Design review of the part built by this model. Coordinates are the model's own, in mm. A direction names the side the tool comes from. Coordinates: 2 decimals unless noted, no trailing zeros. Write each loop counter-clockwise with the first axis right and the second up, starting at its lowest first coordinate (ties: lowest second). Pieces come first, ordered by that corner, then holes. Notation, with made-up numbers: (12, -15.75) -> (58, -15.75) arc R21 cw to (58, 15.25) -> close; hole circle Ø11 at (-30.75, -11). An arc over 180 degrees is marked (long way). Return JSON: item names as keys, results as strings. Group by question number.
from build123d import *

# Parameters (mm, degrees)
BOSS_EXTRUDE1_DEPTH = 50.8
SKETCH2_R           = 2.54
CUT_EXTRUDE1_DEPTH  = 73.955945611
SKETCH3_R           = 3.175
CUT_EXTRUDE2_DEPTH  = 73.955945611
CHAMFER1_SIZE       = 2.54


with BuildPart() as part:
    # Sketch1 → Boss-Extrude1 (new body)
    with BuildSketch(Plane(origin=(0, 0, 0), x_dir=(0, 0, -1), z_dir=(1, 0, 0))):
        with BuildLine():
            Line((0, 1.5875), (0, 50.8))
            Line((0, 50.8), (1.5875, 50.8))
            Line((1.5875, 50.8), (1.5875, 3.175))
            ThreePointArc((1.5875, 3.175), (2.052467985, 2.052467985), (3.175, 1.5875))
            Line((3.175, 1.5875), (12.7, 1.5875))
            Line((12.7, 1.5875), (12.7, 0))
            Line((12.7, 0), (1.5875, 0))
            ThreePointArc((1.5875, 0), (0.464967985, 0.464967985), (0, 1.5875))
        make_face()
    extrude(amount=BOSS_EXTRUDE1_DEPTH)

    # Sketch2 → Cut-Extrude1 (cut, through all)
    with BuildSketch(Plane.XZ):
        with Locations(Location((38.1, -6.35, 0), (0, 0, 270))):
            Circle(SKETCH2_R)
        with Locations(Location((12.7, -6.35, 0), (0, 0, 270))):
            Circle(SKETCH2_R)
    extrude(amount=-CUT_EXTRUDE1_DEPTH, mode=Mode.SUBTRACT)

    # Sketch3 → Cut-Extrude2 (cut, through all)
    with BuildSketch(Plane.XY):
        with Locations((25.4, 25.4)):
            Circle(SKETCH3_R)
    extrude(amount=-CUT_EXTRUDE2_DEPTH, mode=Mode.SUBTRACT)

    # Chamfer1
    chamfer1_edges = [part.edges().sort_by_distance(p)[0] for p in [
        (0, 50.8, -0.79375),
        (50.8, 0.79375, -12.7),
        (50.8, 50.8, -0.79375),
        (0, 0.79375, -12.7),
    ]]
    chamfer(chamfer1_edges, length=CHAMFER1_SIZE)


solid = part.part
Q1. We need section A-A on z = -6.35. Write out the cut boundary in (x, y), plus the area to 3 significant figures.
Q2. Wall thickness on L1, parallel to X at y = 1.1, z = -6.35; L2, parallel to Z at x = 40, y = 17.5; L3, parallel to Y at x = 34, z = -5.5: over which ranges is each line inside the solid? List them lowest first.
Q3. The part is to be moulded in two halves that separate along X. For faces 3 (the flat face through (50.8, 21, -1)), 4 (the cylindrical face through (15.22, 0.78, -6.02)), 5 (the flat face through (1.29, 0.8, -11.45)), say which applies: +X half, -X half, draft (parallel to the pull), parting line (faces both ways), or undercut.
Q4. For P1, Ø1, axis at x = 35, z = -8.5, coming from the +Y side; P2, Ø4.5, axis at x = 38.1, z = -6.35, coming from the -Y side; P3, Ø14.5, axis at x = 17, y = 37, coming from the -Z side, all flat-tipped, find the tip position at first contact; note any pin that passes through.
Q5. We need section D-D on x = 38.1. Write out the cut boundary in (y, z) (1 decimal), plus the area to 3 significant figures.
Q6. We need section C-C on y = 25.4. Write out the cut boundary in (x, z) (1 decimal).
Q7. For faces 1 (the flat face through (25, 22, -1.588)), 2 (the flat face through (25, 50.8, -1)), list the 3-axis set-ups (+Z, -Z, +X, -X, +Y, -Y) from which the entire face can be reached by the end or side of a thin tool; tool diameter is ignored.
Q8. We need section B-B on x = 25.4. Write out the cut boundary in (y, z) (1 decimal), plus the area to 3 significant figures.
Findings below:
{
 "1": {"outline": "(0, 0) -> (10.16, 0) -> (10.16, 1.59) -> (0, 1.59) -> close; (15.24, 0) -> (35.56, 0) -> (35.56, 1.59) -> (15.24, 1.59) -> close; (40.64, 0) -> (50.8, 0) -> (50.8, 1.59) -> (40.64, 1.59) -> close", "area": "64.5 mm^2"},
 "2": {"L1": "x = 0 to 10.16, 15.24 to 35.56, 40.64 to 50.8", "L2": "z = -1.59 to 0", "L3": "y = 0 to 1.59"},
 "3": {"face 3": "+X half", "face 4": "undercut", "face 5": "-X half"},
 "4": {"P1": "stops at y = 1.59", "P2": "passes through", "P3": "stops at z = -1.59"},
 "5": {"outline": "(0, -12.7) -> (1.6, -12.7) -> (1.6, -8.9) -> (0, -8.9) -> close; (0, -3.8) -> (1.6, -3.8) -> (1.6, -3.2) arc R1.6 cw to (3.2, -1.6) -> (50.8, -1.6) -> (50.8, 0) -> (1.6, 0) arc R1.6 ccw to (0, -1.6) -> close", "area": "90.2 mm^2"},
 "6": {"outline": "(0, -1.6) -> (22.2, -1.6) -> (22.2, 0) -> (0, 0) -> close; (28.6, -1.6) -> (50.8, -1.6) -> (50.8, 0) -> (28.6, 0) -> close"},
 "7": {"face 1": "-Z, +X, -X, +Y", "face 2": "+Z, -Z, +X, -X, +Y"},
 "8": {"outline": "(0, -12.7) -> (1.6, -12.7) -> (1.6, -3.2) arc R1.6 cw to (3.2, -1.6) -> (22.2, -1.6) -> (22.2, 0) -> (1.6, 0) arc R1.6 ccw to (0, -1.6) -> close; (28.6, -1.6) -> (50.8, -1.6) -> (50.8, 0) -> (28.6, 0) -> close", "area": "88.2 mm^2"}
}
